```python
from build123d import *

# Parameters (mm, degrees)
RESSALTO_EXTRUS_O1_DEPTH = 40
ESBO_O2_R                = 11
RESSALTO_EXTRUS_O2_DEPTH = 2
ESBO_O3_R                = 2.5
RESSALTO_EXTRUS_O3_DEPTH = 22
ESBO_O4_R                = 1.5
CORTE_EXTRUS_O1_DEPTH    = 15
ESBO_O5_W                = 4.17956517
ESBO_O5_H                = 15
RESSALTO_EXTRUS_O4_DEPTH = 5


with BuildPart() as part:
    # Esboço1 → Ressalto-extrusão1 (new body)
    with BuildSketch(Plane.XY):
        Polygon((-21.15, 16.15), (-16.15, 21.15), (16.15, 21.15), (21.15, 16.15), (21.15, -16.15), (16.15, -21.15), (-16.15, -21.15), (-21.15, -16.15), align=None)
    extrude(amount=RESSALTO_EXTRUS_O1_DEPTH)

    # Esboço2 → Ressalto-extrusão2 (add)
    with BuildSketch(Plane.XY.offset(40)):
        Circle(ESBO_O2_R)
    extrude(amount=RESSALTO_EXTRUS_O2_DEPTH)

    # Esboço3 → Ressalto-extrusão3 (add)
    with BuildSketch(Plane.XY.offset(42)):
        Circle(ESBO_O3_R)
    extrude(amount=RESSALTO_EXTRUS_O3_DEPTH)

    # Esboço4 → Corte-extrusão1 (cut)
    with BuildSketch(Plane.XY.offset(40)):
        with Locations((15.5, -15.5)):
            Circle(ESBO_O4_R)
        with Locations((15.5, 15.5)):
            Circle(ESBO_O4_R)
        with Locations((-15.5, -15.5)):
            Circle(ESBO_O4_R)
        with Locations((-15.5, 15.5)):
            Circle(ESBO_O4_R)
    extrude(amount=-CORTE_EXTRUS_O1_DEPTH, mode=Mode.SUBTRACT)

    # Esboço5 → Ressalto-extrusão4 (add)
    with BuildSketch(Plane(origin=(21.15, 0, 0), x_dir=(0, 0, -1), z_dir=(1, 0, 0))):
        with Locations((-2.436524566, 0)):
            Rectangle(ESBO_O5_W, ESBO_O5_H)
    extrude(amount=RESSALTO_EXTRUS_O4_DEPTH)


solid = part.part
```
Work out the finished part from the listing and answer in its coordinate system (mm). A direction names the side the tool comes from. Round coordinates to 2 decimals unless told otherwise and drop trailing zeros. Loops run counter-clockwise (first coordinate to the right, second up) from the corner with the lowest first, then second, coordinate; pieces in that order, holes last. Notation, with made-up numbers: M 37.5,60 L 69.5,60 A31 ccw 69.5,87 Z; hole C -39.75,61 d9. An arc over 180 degrees is marked long. Use CSV: the item, a comma, the result in double quotes.
Q1. Consider L1, parallel to Y at x = 15.5, z = 33.75; L2, parallel to Y at x = 15, z = 30; L3, parallel to Z at x = 12.5, y = 8.5. Determine where each line is inside the solid, lowest interval first.
Determined:
L1,"-21.15 to -17, -14 to 14, 17 to 21.15"
L2,"-21.15 to -16.91, -14.09 to 14.09, 16.91 to 21.15"
L3,"0 to 40"
Q2. Each of these flat-tipped pins is pushed along its axis until it touches: pin 1 (1.8 mm diameter, centred on x = -15.5, y = -15.5, fed in from +Z); pin 2 (12.5 mm diameter, centred on x = 5.5, y = -9, fed in from +Z); pin 3 (4 mm diameter, centred on x = 23.5, y = 0.5, fed in from +Z); pin 4 (2 mm diameter, centred on y = 5, z = 45, fed in from -X). Where does it stop, or does it pass through?
Determined:
pin 1,"z = 25"
pin 2,"z = 42"
pin 3,"z = 4.53"
pin 4,"through"
Q3. The mould has two halves that part along X. Classify faces 1 (the cylindrical face through (14, -15.43, 32.61)), 2 (the flat face through (-9, -9, 40)), 3 (the flat face through (-18.6, -18.7, 19.7)): pulls with the +X half, pulls with the -X half, needs draft (parallel to the pull), parting line crosses it, or undercut.
Determined:
face 1,"undercut"
face 2,"needs draft"
face 3,"pulls with the -X half"
Q4. Section A-A, the plane z = 29.5 is taken. Determine the outline of the cut face in (x, y).
Determined:
outline,"M -21.15,-16.15 L -16.15,-21.15 L 16.15,-21.15 L 21.15,-16.15 L 21.15,16.15 L 16.15,21.15 L -16.15,21.15 L -21.15,16.15 Z; hole C -15.5,-15.5 d3; hole C -15.5,15.5 d3; hole C 15.5,-15.5 d3; hole C 15.5,15.5 d3"
Q5. Section B-B, the plane y = -5.5 is taken. Determine the outline of the cut face in (x, z).
Determined:
outline,"M -21.15,0 L 21.15,0 L 21.15,0.35 L 26.15,0.35 L 26.15,4.53 L 21.15,4.53 L 21.15,40 L 9.53,40 L 9.53,42 L -9.53,42 L -9.53,40 L -21.15,40 Z"
Q6. Section D-D, the plane z = 21.5 is taken. Determine the outline of the cut face in (x, y).
Determined:
outline,"M -21.15,-16.15 L -16.15,-21.15 L 16.15,-21.15 L 21.15,-16.15 L 21.15,16.15 L 16.15,21.15 L -16.15,21.15 L -21.15,16.15 Z"
Q7. Section C-C, the plane x = 1 is taken. Determine the outline of the cut face in (y, z).
Determined:
outline,"M -21.15,0 L 21.15,0 L 21.15,40 L 10.95,40 L 10.95,42 L 2.29,42 L 2.29,64 L -2.29,64 L -2.29,42 L -10.95,42 L -10.95,40 L -21.15,40 Z"
Q8. A tool of negligible diameter and unlimited length cuts with its end or side. For faces 4 (the cylindrical face through (-0.54, -2.44, 52.85)), 5 (the flat face through (24, 0, 0.347)), 6 (the flat face through (0, 21.15, 20)), from which of +Z, -Z, +X, -X, +Y, -Y can it reach the whole face along a straight path? Write none if from no direction.
Determined:
face 4,"+Z"
face 5,"-Z, +X, +Y, -Y"
face 6,"+Z, -Z, +X, -X, +Y"
